Input: part model. Units: mm. Frame: model coordinates. A direction names the side the tool comes from. Coordinates: 2 decimals unless noted, no trailing zeros. Write each loop counter-clockwise with the first axis right and the second up, starting at its lowest first coordinate (ties: lowest second). Pieces come first, ordered by that corner, then holes. Notation, with made-up numbers: (57.25, -38) - (80.25, -38) arc R27 ccw to (80.25, -18) - close; hole circle Ø7 at (17, 55.25). An arc over 180 degrees is marked (long way). Use CSV: the item, a comma, the result in double quotes.
```python
from build123d import *

# Parameters (mm, degrees)
PAD_DEPTH        = 25
SKETCH001_W      = 84
SKETCH001_H      = 19
SKETCH002_W      = 54
SKETCH002_H      = 7
SKETCH003_W      = 88.531874
SKETCH003_H      = 19
POCKET_DEPTH     = 5
SKETCH004_W      = 90
SKETCH004_H      = 105
PAD001_DEPTH     = 3
HOLE_D           = 4.5
HOLE_DEPTH       = 25
HOLE_CSINK_D     = 9
HOLE_CSINK_ANGLE = 90


with BuildPart() as part:
    # Sketch → Pad (new body)
    with BuildSketch(Plane.XY):
        Polygon((-45, 70), (-45, -21.531874), (-45, -70), (15, -70), (45, 7.838913), (45, 70), align=None)
    extrude(amount=PAD_DEPTH)

    # Sketch001 (on Face6 of Pad) → SubtractiveLoft section 0
    with BuildSketch(Plane(origin=(0, 70, 0), x_dir=(-1, 0, 0), z_dir=(0, 1, 0))):
        with Locations((0, 12.5)):
            Rectangle(SKETCH001_W, SKETCH001_H)
    # Sketch002 (on Face3 of Pad) → SubtractiveLoft section 1
    with BuildSketch(Plane.XZ.offset(70)):
        with Locations((-15, 12.5)):
            Rectangle(SKETCH002_W, SKETCH002_H)
    loft(mode=Mode.SUBTRACT)

    # Sketch003 (on Face1 of SubtractiveLoft) → Pocket (cut)
    with BuildSketch(Plane(origin=(-45, 0, 0), x_dir=(0, -1, 0), z_dir=(-1, 0, 0))):
        with Locations((-22.734063, 12.5)):
            Rectangle(SKETCH003_W, SKETCH003_H)
    extrude(amount=-POCKET_DEPTH, mode=Mode.SUBTRACT)

    # Sketch004 (on Face8 of Pocket) → Pad001 (join)
    with BuildSketch(Plane(origin=(0, 70, 0), x_dir=(-1, 0, 0), z_dir=(0, 1, 0))):
        with Locations((0, 12.5)):
            Rectangle(SKETCH004_W, SKETCH004_H)
    extrude(amount=PAD001_DEPTH)

    # Hole
    with Locations(Plane.XZ.offset(-70)):
        with Locations((-37.5, 57.5), (-37.5, -32.5)):
            hole = CounterSinkHole(HOLE_D / 2, HOLE_CSINK_D / 2, depth=HOLE_DEPTH, counter_sink_angle=HOLE_CSINK_ANGLE)

    # Mirrored: Hole across Sketch005 V_Axis
    add(hole.mirror(Plane(origin=(0, 70, 0), x_dir=(0, -1, 0), z_dir=(1, 0, 0))), mode=Mode.SUBTRACT)


solid = part.part
```
(1) Cut plane A-A on z = -32.5. Return loops of the section in (x, y), and give its area (3 significant figures).
Check values:
outline,"(-45, 70) - (-42, 70) - (-39.75, 72.25) - (-39.75, 73) - (-45, 73) - close; (-35.25, 72.25) - (-33, 70) - (33, 70) - (35.25, 72.25) - (35.25, 73) - (-35.25, 73) - close; (39.75, 72.25) - (42, 70) - (45, 70) - (45, 73) - (39.75, 73) - close"
area,"233 mm^2"
(2) Pin query (flat end, axial travel): pin 1 Ø8 at (x, y) = (-13.5, 26) entering from +Z; pin 2 Ø1.5 at (x, y) = (-43.5, 36) entering from -Z; pin 3 Ø1.2 at (y, z) = (14.5, 4.5) entering from -X. Return the tip coordinate at first contact, or that it passes through.
Check values:
pin 1,"z = 25"
pin 2,"z = 0"
pin 3,"x = -40"
(3) Cut plane B-B on x = 37.5. State how many separate pieces and enclosed holes the cut face has, and give its area (3 significant figures).
Check values:
separate pieces,"3"
enclosed holes,"1"
area,"1,940 mm^2"
(4) Cut plane D-D on z = -5.5. Return loops of the section in (x, y), and give its area (3 significant figures).
Check values:
outline,"(-45, 70) - (45, 70) - (45, 73) - (-45, 73) - close"
area,"270 mm^2"
(5) Ray query, probe 1 along Z at (x, y) = (37.5, 72.4); probe 2 along X at (y, z) = (72.45, 57.5); probe 3 along X at (y, z) = (72, -32). Return the intervals inside material, ascending. Write a range as from..to.
Check values:
probe 1,"-40..-34.75, -30.25..55.25, 59.75..65"
probe 2,"-45..-39.75, -35.25..35.25, 39.75..45"
probe 3,"-45..-39.95, -35.05..35.05, 39.95..45"
(6) Draft query along X for faces 1 (the flat face through (45, 45, 12)), 2 (the cylindrical face through (38.71, 72.63, -30.603)), 3 (the flat face through (-45, -4, 1)). Return one class per face: pulls with the +X half, pulls with the -X half, needs draft (parallel to the pull), parting line crosses it, or undercut.
Check values:
face 1,"pulls with the +X half"
face 2,"undercut"
face 3,"pulls with the -X half"
(7) Reachability of faces 4 (the flat face through (-40, 14, 4)), 5 (the flat face through (-15, -70, 18)), 6 (the flat face through (1, 70, 45)), 7 (the flat face through (-1, 1, 0)), 8 (the conical face through (-38.77, 72.14, 59.49)) from +Z, -Z, +X, -X, +Y, -Y: full face, straight path, thin tool, end or side. Return the list, or none.
Check values:
face 4,"-X"
face 5,"+Z, -Z, +X, -X, -Y"
face 6,"+Z, +X, -X, -Y"
face 7,"-Z, +X, -X, -Y"
face 8,"-Y"
